Autodesk Inventor part; units mm, degrees
ref_plane "YZ Plane" through (0, 0, 0) normal (1, 0, 0) x (0, 1, 0)
ref_plane "XZ Plane" through (0, 0, 0) normal (0, 1, 0) x (-1, 0, 0)
ref_plane "XY Plane" through (0, 0, 0) normal (0, 0, 1) x (1, 0, 0)
sketch "Sketch1" plane through (0, 0, 0) normal (0, 0, 1) x (1, 0, 0)
  circle A0 centre (0, 0) radius 28.575
  dimension "d0" = 57.15
extrude "Extrusion1" add sketch "Sketch1" along normal blind 4.572
sketch "Sketch2" plane through (0, 0, 4.572) normal (0, 0, 1) x (1, 0, 0)
  circle A0 centre (0, 0) radius 28.575
  circle A1 centre (0, 0) radius 12.1666
  dimension "d3" = 24.3332
extrude "Extrusion2" add sketch "Sketch2" along normal blind 20.828 contours A1
sketch "Sketch3" plane through (0, 0, 25.4) normal (0, 0, 1) x (1, 0, 0)
  circle A0 centre (0, 0) radius 12.1666
  circle A1 centre (0, 0) radius 6.35
  line L0 (-1.5875, 7.7359) -> (1.5875, 7.7359)
  line L1 (1.5875, 7.7359) -> (1.5875, 4.5609)
  line L2 (1.5875, 4.5609) -> (-1.5875, 4.5609)
  line L3 (-1.5875, 4.5609) -> (-1.5875, 7.7359)
  point P0 (0, 7.7359)
  point P1 (-1.5875, 6.1484)
  dimension "d6" = 12.7
  dimension "d7" = 3.175
  dimension "d8" = 3.175
extrude "Extrusion3" cut sketch "Sketch3" against normal through all contours A1 L3 L2 L1 | L1 L2 L3 A1 | A1 L3 L0 L1
properties part number "Hub 500 key"
Could you check a few things on this model? Use its own coordinates, in mm. A direction names the side the tool comes from. Coordinates: 2 decimals unless noted, no trailing zeros. Loops run counter-clockwise (first coordinate to the right, second up) from the corner with the lowest first, then second, coordinate; pieces in that order, holes last. Notation, with made-up numbers: (14.25, -10) -> (68.25, -10) arc R13 cw to (68.25, 5) -> close; hole circle Ø2 at (-18, -27.5). An arc over 180 degrees is marked (long way). Answer in a Markdown table with one row per item.
(1) Will these pins go through, and if not, where does the flat tip stop? pin 1 Ø2.5 at (x, z) = (0.5, 13.5) entering from -Y; pin 2 Ø1.3 at (y, z) = (7, 10) entering from -X; pin 3 Ø3 at (x, z) = (5, 10) entering from -Y.
Results found:
| item | result |
|---|---|
| pin 1 | stops at y = -12.17 |
| pin 2 | stops at x = -10.38 |
| pin 3 | stops at y = -11.65 |
(2) If I drill on probe 1 along Y at (x, z) = (0, 16); probe 2 along Z at (x, y) = (-16.5, 3); probe 3 along X at (y, z) = (7, 14), over which ranges is the centre line in solid material (lowest first)?
Results found:
| item | result |
|---|---|
| probe 1 | y = -12.17 to -6.35, 7.74 to 12.17 |
| probe 2 | z = 0 to 4.57 |
| probe 3 | x = -9.95 to -1.59, 1.59 to 9.95 |
(3) Thinking about a two-plate mould opening in X: for faces 1 (the face through (-2, -12, 15)), 2 (the face through (1.588, 7, 13)), 3 (the face through (5, -5, 25.4)), which applies, released by +X, released by -X, zero draft, split by the parting line, or undercut?
Results found:
| item | result |
|---|---|
| face 1 | split by the parting line |
| face 2 | undercut |
| face 3 | zero draft |
(4) Imagine slicing it at B-B (x = 0). List the corners of the cut face in (y, z) for me (3 decimals).
Results found:
| item | result |
|---|---|
| outline | (-28.575, 0) -> (-6.35, 0) -> (-6.35, 25.4) -> (-12.167, 25.4) -> (-12.167, 4.572) -> (-28.575, 4.572) -> close; (7.736, 0) -> (28.575, 0) -> (28.575, 4.572) -> (12.167, 4.572) -> (12.167, 25.4) -> (7.736, 25.4) -> close |
(5) Imagine slicing it at D-D (y = 10). List the corners of the cut face in (x, z) for me, plus the area to 3 significant figures.
Results found:
| item | result |
|---|---|
| outline | (-26.77, 0) -> (26.77, 0) -> (26.77, 4.57) -> (6.93, 4.57) -> (6.93, 25.4) -> (-6.93, 25.4) -> (-6.93, 4.57) -> (-26.77, 4.57) -> close |
| area | 533 mm^2 |
(6) Imagine slicing it at C-C (z = 16.5). List the corners of the cut face in (x, y) for me.
Results found:
| item | result |
|---|---|
| outline | circle Ø24.33 at (0, 0); hole (-1.59, 6.15) arc R6.35 ccw (long way) to (1.59, 6.15) -> (1.59, 7.74) -> (-1.59, 7.74) -> close |
(7) For faces 4 (the face through (-1.588, 7, 13)), 5 (the face through (-7, 0, 0)), 6 (the face through (12, -6, 4.572)), which set-ups out of +Z, -Z, +X, -X, +Y, -Y let a thin tool reach every point of the face, with its end or its side?
Results found:
| item | result |
|---|---|
| face 4 | +Z, -Z |
| face 5 | -Z, +X, -X, +Y, -Y |
| face 6 | +Z |
(8) Imagine slicing it at A-A (y = 0). List the corners of the cut face in (x, z) for me (3 decimals), plus the area to 3 significant figures.
Results found:
| item | result |
|---|---|
| outline | (-28.575, 0) -> (-6.35, 0) -> (-6.35, 25.4) -> (-12.167, 25.4) -> (-12.167, 4.572) -> (-28.575, 4.572) -> close; (6.35, 0) -> (28.575, 0) -> (28.575, 4.572) -> (12.167, 4.572) -> (12.167, 25.4) -> (6.35, 25.4) -> close |
| area | 446 mm^2 |
